Could you check a few things on this model? Use its own coordinates, in mm. Face numbers are marked on the shaded views. A direction names the side the tool comes from. Coordinates: 2 decimals unless noted, no trailing zeros. Loops run counter-clockwise (first coordinate to the right, second up) from the corner with the lowest first, then second, coordinate; pieces in that order, holes last.
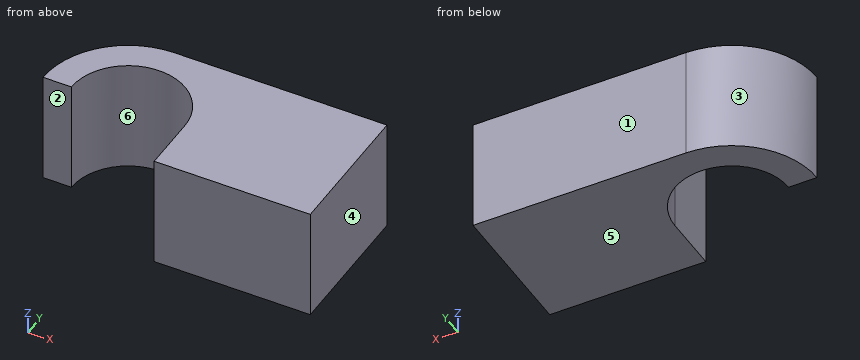
from build123d import *

# Parameters (mm, degrees)
F1_DEPTH = 4


with BuildPart() as f1:
    # F0 (on Top) → F1 (new body, symmetric)
    with BuildSketch(Plane.XY):
        with BuildLine():
            ThreePointArc((-4, 0), (0, 4), (4, 0))
            Line((4, 0), (4, -4))
            Line((4, -4), (15, -4))
            Line((15, -4), (15, 6))
            Line((15, 6), (0, 6))
            ThreePointArc((0, 6), (-4.242641, 4.242641), (-6, 0))
            Line((-6, 0), (-4, 0))
        make_face()
    extrude(amount=F1_DEPTH, both=True)


solid = f1.part
(1) I need wall thicknesses on probe 1 along X at (y, z) = (-1.5, 2); probe 2 along X at (y, z) = (1.5, 2.5); probe 3 along X at (y, z) = (3, 0.5). Which ranges of each line are inside material? Lowest first, please.
Answers:
probe 1: x = 4 to 15
probe 2: x = -5.81 to -3.71, 3.71 to 15
probe 3: x = -5.2 to -2.65, 2.65 to 15
(2) Which directions (+Z, -Z, +X, -X, +Y, -Y) give clear straight access to the entire face, cutting with the end or side of a thin tool? Please do the marked faces 1 and 2.
Answers:
face 1: +Z, -Z, +X, -X, +Y
face 2: +Z, -Z, -X, -Y
(3) Imagine slicing it at A-A, the plane z = 1.5. Write out the boundary of the cut face in (x, y).
Answers:
outline: (-6, 0) - (-4, 0) arc R4 cw to (4, 0) - (4, -4) - (15, -4) - (15, 6) - (0, 6) arc R6 ccw to start
(4) Imagine slicing it at B-B, the plane y = 3.25. Write out the boundary of the cut face in (x, z), and give its area (3 significant figures).
Answers:
outline: (-5.04, -4) - (-2.33, -4) - (-2.33, 4) - (-5.04, 4) - close; (2.33, -4) - (15, -4) - (15, 4) - (2.33, 4) - close
area: 123 mm2
(5) Imagine slicing it at D-D, the plane x = -1.75. Write out the boundary of the cut face in (y, z), and give its area (3 significant figures).
Answers:
outline: (3.6, -4) - (5.74, -4) - (5.74, 4) - (3.6, 4) - close
area: 17.1 mm2
(6) Imagine slicing it at C-C, the plane y = -0.25. Write out the boundary of the cut face in (x, z).
Answers:
outline: (4, -4) - (15, -4) - (15, 4) - (4, 4) - close
(7) For pin 1 (1.2 mm diameter, centred on y = -1.5, z = -1.5, fed in from -X); pin 2 (1.5 mm diameter, centred on y = 1, z = 1.5, fed in from -X); pin 3 (1 mm diameter, centred on y = 3, z = 3, fed in from -X); pin 4 (3 mm diameter, centred on x = -3, y = 1.5, fed in from -Z), each with a flat end and sliding along its axis, tell me the tip position at first contact or that it passes through.
Answers:
pin 1: stops at x = 4
pin 2: stops at x = -5.99
pin 3: stops at x = -5.45
pin 4: stops at z = -4
(8) We'd pull the mould along X, two halves only. Please class the marked faces 3, 4, 5 and 6: +X half, -X half, draft (parallel to the pull), parting line (faces both ways), or undercut.
Answers:
face 3: -X half
face 4: +X half
face 5: draft
face 6: undercut
